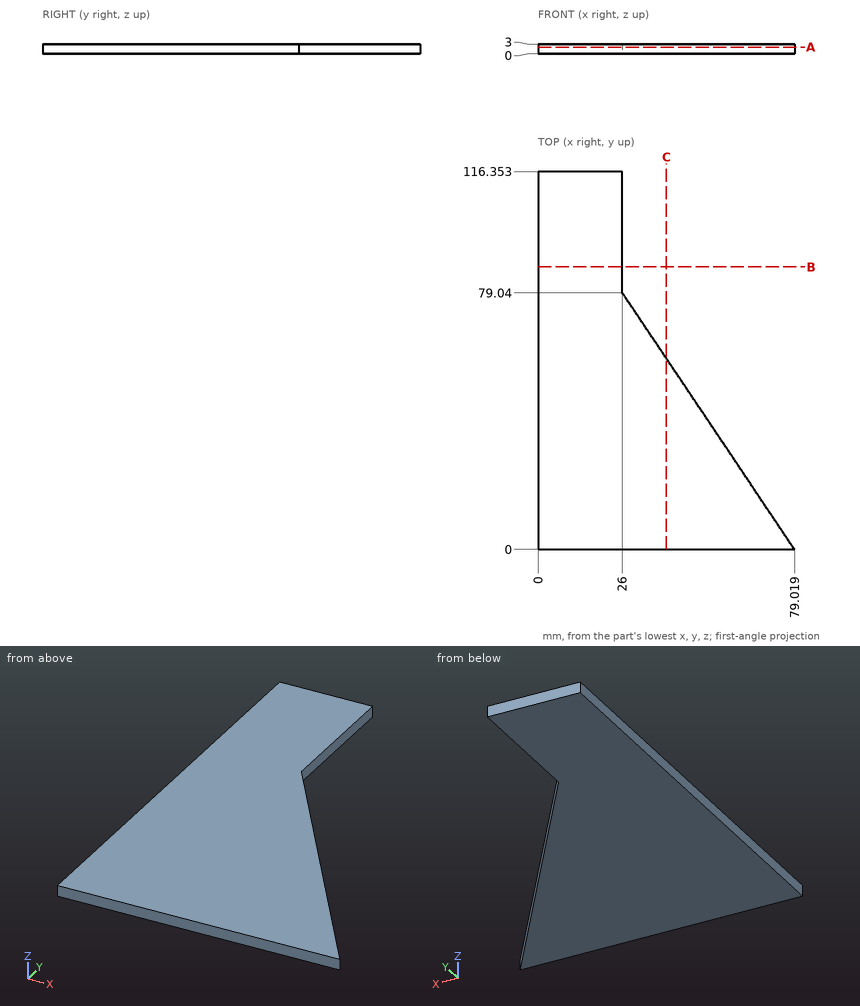
Can you work these out from the drawing? Everything is in mm from the part's minimum corner. Give positions to 0.01 mm unless a question says otherwise; leave off trailing zeros. Order: outer loops, then holes, each group sorted by start corner. A loop starts at its lowest first (then second) coordinate and runs counter-clockwise, first axis right, second up. Notation, with made-up numbers: (72.5, 2.25) -> (125.5, 2.25) arc R10 ccw to (125.5, 19.25) -> close; hole circle Ø9 at (59, 73). An arc over 180 degrees is marked (long way). Return JSON: item names as keys, results as strings.
1. Imagine slicing it at B-B on y = 87. List the corners of the cut face in (x, z) for me.
Answer list:
{"outline": "(0, 0) -> (26, 0) -> (26, 3) -> (0, 3) -> close"}
2. I need wall thicknesses on line 1 (X direction, y = 108.5, z = 0.25); line 2 (Y direction, x = 75.5, z = 2.1) (1 decimal); line 3 (X direction, y = 56, z = 2.55) (1 decimal). Which ranges of each line are inside material? Lowest first, please. Write a range as from..to.
Answer list:
{"line 1": "x = 0..26", "line 2": "y = 0..5.2", "line 3": "x = 0..41.5"}
3. Imagine slicing it at A-A on z = 2.05. List the corners of the cut face in (x, y) for me.
Answer list:
{"outline": "(0, 0) -> (79.02, 0) -> (26, 79.04) -> (26, 116.35) -> (0, 116.35) -> close"}
4. Imagine slicing it at C-C on x = 39.5. List the corners of the cut face in (y, z) for me, then the cut area to 3 significant figures.
Answer list:
{"outline": "(0, 0) -> (58.91, 0) -> (58.91, 3) -> (0, 3) -> close", "area": "177 mm2"}
5. For pin 1 Ø1.5 at (y, z) = (54.5, 1.5) entering from +X; pin 2 Ø0.9 at (y, z) = (99.5, 1) entering from +X, each with a flat end and sliding along its axis, tell me the tip position at first contact or that it passes through.
Answer list:
{"pin 1": "stops at x = 42.96", "pin 2": "stops at x = 26"}
